Read the model definition and answer for the solid it produces. Units are mm, in the model's axes. Face numbers are marked on the shaded views. A direction names the side the tool comes from. Coordinates: 2 decimals unless noted, no trailing zeros. Write each loop counter-clockwise with the first axis right and the second up, starting at its lowest first coordinate (ties: lowest second). Pieces come first, ordered by that corner, then holes. Notation, with made-up numbers: (-38.5, -15) - (-19.5, -15) arc R22 cw to (-19.5, 6) - close; hole circle Ø1 at (52, -7). An arc over 180 degrees is marked (long way). Return JSON: item names as keys, results as strings.
```python
from build123d import *

# Parameters (mm, degrees)
EXTRU_MINCE1_DEPTH      = 50
ESQUISSE2_W             = 36
ESQUISSE2_H             = 3.5
ENL_V_MAT_EXTRU_1_DEPTH = 100


with BuildPart() as part:
    # Esquisse1 → Extru.-Mince1 (new body)
    with BuildSketch(Plane.XY):
        Polygon((-50, 50), (-50, 0), (0, 0), (0, 100), (6.6, 100), (6.6, 0), (56.6, 0), (56.6, 50), (46.6, 50), (46.6, 10), (16.6, 10), (16.6, 110), (-10, 110), (-10, 10), (-40, 10), (-40, 50), align=None)
    extrude(amount=EXTRU_MINCE1_DEPTH)

    # Esquisse2 → Enlèv. mat.-Extru.1 (cut)
    with BuildSketch(Plane(origin=(0, 10, 0), x_dir=(1, 0, 0), z_dir=(0, 1, 0))):
        with Locations((-25.454999668, -5.571109307)):
            Rectangle(ESQUISSE2_W, ESQUISSE2_H)
        with Locations((-25.454999668, -44.515273736)):
            Rectangle(ESQUISSE2_W, ESQUISSE2_H)
        with Locations((31.312560908, -5.571109307)):
            Rectangle(ESQUISSE2_W, ESQUISSE2_H)
        with Locations((31.312560908, -44.515273736)):
            Rectangle(ESQUISSE2_W, ESQUISSE2_H)
    extrude(amount=ENL_V_MAT_EXTRU_1_DEPTH, mode=Mode.SUBTRACT)


solid = part.part
```
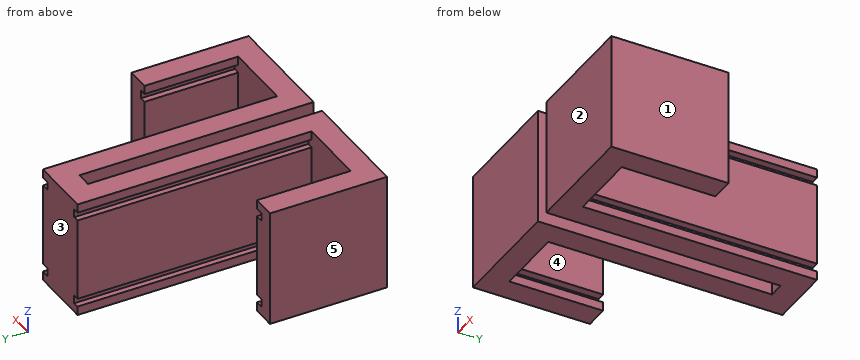
(1) Determine the mould class of the marked faces 1, 2 and 3 for opening direction Y: +Y half, -Y half, draft (parallel to the pull), parting line (faces both ways), or undercut.
Answer:
{"face 1": "draft", "face 2": "-Y half", "face 3": "+Y half"}
(2) Which of the six approach directions +Z, -Z, +X, -X, +Y, -Y give full straight-line access (tool end or side, diameter ignored) to the marked faces 4 and 5?
Answer:
{"face 4": "+Z, -Z, +Y", "face 5": "+Z, -Z, -X, +Y, -Y"}
(3) A cutting plane is placed at C-C (y = 29.5). State how many separate pieces and enclosed holes the cut face has, and give its area (3 significant figures).
Answer:
{"separate pieces": "4", "enclosed holes": "0", "area": "1,920 mm²"}
(4) A cutting plane is placed at D-D (x = 18). Determine the outline of the cut face in (y, z).
Answer:
{"outline": "(0, 0) - (10, 0) - (10, 50) - (0, 50) - close"}
(5) A cutting plane is placed at B-B (z = 23). Determine the outline of the cut face in (x, y).
Answer:
{"outline": "(-50, 0) - (0, 0) - (0, 100) - (6.6, 100) - (6.6, 0) - (56.6, 0) - (56.6, 50) - (46.6, 50) - (46.6, 10) - (16.6, 10) - (16.6, 110) - (-10, 110) - (-10, 10) - (-40, 10) - (-40, 50) - (-50, 50) - close"}
(6) Straight lines are drawn through the part: line 1 (X direction, y = 34, z = 15.5); line 2 (X direction, y = 52, z = 26.5); line 3 (Z direction, x = -41, y = 47). For each, find the intervals that lie inside material, in ascending order. Write a range as from..to.
Answer:
{"line 1": "-50..-40, -10..0, 6.6..16.6, 46.6..56.6", "line 2": "-10..0, 6.6..16.6", "line 3": "0..3.82, 7.32..42.77, 46.27..50"}
(7) A cutting plane is placed at A-A (y = 75). Determine the outline of the cut face in (x, z) (3 decimals), and give its area (3 significant figures).
Answer:
{"outline": "(-10, 0) - (0, 0) - (0, 50) - (-10, 50) - (-10, 46.265) - (-7.455, 46.265) - (-7.455, 42.765) - (-10, 42.765) - (-10, 7.321) - (-7.455, 7.321) - (-7.455, 3.821) - (-10, 3.821) - close; (6.6, 0) - (16.6, 0) - (16.6, 3.821) - (13.313, 3.821) - (13.313, 7.321) - (16.6, 7.321) - (16.6, 42.765) - (13.313, 42.765) - (13.313, 46.265) - (16.6, 46.265) - (16.6, 50) - (6.6, 50) - close", "area": "959 mm²"}
(8) Flat-ended cylindrical pins translate along their axes: P1, Ø5, axis at x = 54, z = 20.5, coming from the +Y side; P2, Ø10.5, axis at y = 75, z = 31.5, coming from the +X side; P3, Ø1, axis at y = 65, z = 5.5, coming from the +X side. Find the tip coordinate at first contact, or state that the pin passes through.
Answer:
{"P1": "y = 50", "P2": "x = 16.6", "P3": "x = 13.31"}
